Work out the finished part from the listing and answer in its coordinate system (mm). Face numbers are marked on the shaded views. A direction names the side the tool comes from. Give positions to 0.01 mm unless a question says otherwise; leave off trailing zeros. Loops run counter-clockwise (first coordinate to the right, second up) from the corner with the lowest first, then second, coordinate; pieces in that order, holes last.
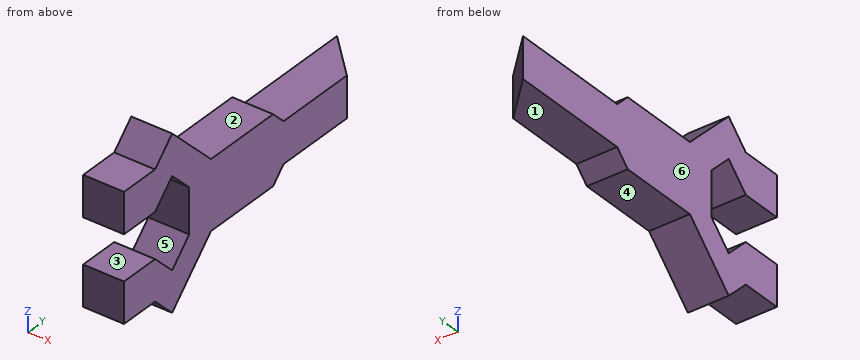
from build123d import *

# Parameters (mm, degrees)
BOSS_EXTRUDE1_DEPTH = 10
BOSS_EXTRUDE2_DEPTH = 5


with BuildPart() as part:
    # Sketch1 → Boss-Extrude1 (new body)
    with BuildSketch(Plane(origin=(0, 0, 0), x_dir=(0, 0, -1), z_dir=(1, 0, 0))):
        Polygon((5.5, 5.5), (11, 0), (5.5, -5.5), (5.5, -15.5), (15.399494937, -15.5), (15.399494937, -5.5), (20.899494937, 0), (8.399494937, 12.5), (8.399494937, 32.5), (0, 40.899494937), (-8.399494937, 32.5), (-8.399494937, 12.5), (-20.899494937, 0), (-15.399494937, -5.5), (-15.399494937, -15.5), (-5.5, -15.5), (-5.5, -5.5), (-11, 0), (-5.5, 5.5), align=None)
    extrude(amount=BOSS_EXTRUDE1_DEPTH)

    # Sketch2 → Boss-Extrude2 (add, symmetric)
    with BuildSketch(Plane.XY):
        Polygon((0, 6.25), (0, 66.25), (10, 56.25), (10, 6.25), align=None)
    extrude(amount=BOSS_EXTRUDE2_DEPTH, both=True)


solid = part.part
Item 1: Find section C-C, the plane z = 10. Write down the section's boundary in (x, y), plus the area to 3 significant figures.
Item 2: Determine the mould class of the marked faces 4, 5 and 6 for opening direction Z: released by +Z, released by -Z, zero draft, split by the parting line, or undercut.
Item 3: Find section B-B, the plane y = -1. Write down the section's boundary in (x, z), plus the area to 3 significant figures.
Item 4: Consider line 1 (Z direction, x = 1, y = -9.5); line 2 (Z direction, x = 1.75, y = 51.5); line 3 (Y direction, x = 2.75, z = -8). Determine where each line is inside the solid, lowest interval first.
Item 5: Find section D-D, the plane y = 39. Write down the section's boundary in (x, z).
Item 6: For the marked faces 1, 2 and 3, determine the directions among +Z, -Z, +X, -X, +Y, -Y from which every point of the face is accessible in a straight line to the end or side of a thin tool.
Item 7: Flat-ended cylindrical pins translate along their axes: pin 1 Ø3 at (x, y) = (1.5, 33.5) entering from +Z; pin 2 Ø3 at (x, y) = (5, -9.5) entering from -Z; pin 3 Ø1.5 at (x, z) = (2.5, -2) entering from +Y. Find the tip coordinate at first contact, or state that the pin passes through.
Item 8: Find section A-A, the plane x = 1.25. Write down the section's boundary in (y, z), plus the area to 3 significant figures.
Ans:
1. outline: (0, -15.5) - (10, -15.5) - (10, -1) - (0, -1) - close; (0, 1) - (10, 1) - (10, 10.9) - (0, 10.9) - close
1. area: 244 mm2
2. face 4: released by -Z
2. face 5: undercut
2. face 6: zero draft
3. outline: (0, -19.9) - (10, -19.9) - (10, -10) - (0, -10) - close; (0, 10) - (10, 10) - (10, 19.9) - (0, 19.9) - close
3. area: 198 mm2
4. line 1: z = -15.4 to -5.5, 5.5 to 15.4
4. line 2: z = -5 to 5
4. line 3: y = -15.5 to -3, 3 to 32.9
5. outline: (0, -5) - (10, -5) - (10, 5) - (0, 5) - close
6. face 1: -Z, +X, -X, +Y
6. face 2: +Z, +X, -X, +Y
6. face 3: +X, -X, -Y
7. pin 1: stops at z = 8.4
7. pin 2: stops at z = -15.4
7. pin 3: stops at y = 64.5
8. outline: (-15.5, -15.4) - (-5.5, -15.4) - (0, -20.9) - (12.5, -8.4) - (32.5, -8.4) - (35.9, -5) - (65, -5) - (65, 5) - (35.9, 5) - (32.5, 8.4) - (12.5, 8.4) - (0, 20.9) - (-5.5, 15.4) - (-15.5, 15.4) - (-15.5, 5.5) - (-5.5, 5.5) - (0, 11) - (5.5, 5.5) - (5.5, -5.5) - (0, -11) - (-5.5, -5.5) - (-15.5, -5.5) - close
8. area: 1,250 mm2
